from build123d import *

# Parameters (mm, degrees)
CYLINDER_R     = 10
CYLINDER_DEPTH = 40
BOX_W          = 30
BOX_H          = 24
BOX_DEPTH      = 40


with BuildPart() as cilindro:
    # Cylinder → Cylinder (new body)
    with BuildSketch(Plane(origin=(11, 12, -16), x_dir=(1, 0, 0), z_dir=(0, 0, 1))):
        Circle(CYLINDER_R)
    extrude(amount=CYLINDER_DEPTH)


with BuildPart() as cut:
    # Box → Box (new body)
    with BuildSketch(Plane(origin=(-1, 0, -12), x_dir=(1, 0, 0), z_dir=(0, 0, 1))):
        with Locations((15, 12)):
            Rectangle(BOX_W, BOX_H)
    extrude(amount=BOX_DEPTH)

    # Cut: cut Cilindro
    add(cilindro.part, mode=Mode.SUBTRACT)


solid = cut.part
Could you check a few things on this model? Use its own coordinates, in mm. A direction names the side the tool comes from. Give positions to 0.01 mm unless a question says otherwise; leave off trailing zeros. Order: outer loops, then holes, each group sorted by start corner. A loop starts at its lowest first (then second) coordinate and runs counter-clockwise, first axis right, second up. Notation, with made-up numbers: M 36.5,35.25 L 68.5,35.25 A22 ccw 68.5,47.25 Z; hole C 67,-39 d5. An arc over 180 degrees is marked long. One line per question, with ' | ' between items.
1. I want a section at C-C (x = 3). List the corners of the cut face in (y, z) for me, and give its area (3 significant figures).
Results:
outline: M 0,-12 L 6,-12 L 6,24 L 18,24 L 18,-12 L 24,-12 L 24,28 L 0,28 Z | area: 528 mm²
2. For faces 4 (the face through (11, 12, 24)), 5 (the face through (20, 18, -12)), which set-ups out of +Z, -Z, +X, -X, +Y, -Y let a thin tool reach every point of the face, with its end or its side?
Results:
face 4: -Z | face 5: -Z, +X, -X, +Y, -Y
3. We'd pull the mould along X, two halves only. Please class faces 1 (the face through (29, 12, 8)), 2 (the face through (14, 12, 28)), 3 (the face through (3, 6, 6)): +X half, -X half, draft (parallel to the pull), parting line (faces both ways), or undercut.
Results:
face 1: +X half | face 2: draft | face 3: undercut
4. I want a section at B-B (y = 12). List the corners of the cut face in (x, z) for me.
Results:
outline: M -1,-12 L 1,-12 L 1,24 L 21,24 L 21,-12 L 29,-12 L 29,28 L -1,28 Z
5. I want a section at A-A (z = 4.5). List the corners of the cut face in (x, y) for me.
Results:
outline: M -1,0 L 29,0 L 29,24 L -1,24 Z; hole C 11,12 d20
6. I'm going to push a flat-ended pin straight in: pin 1 (1.5 mm diameter, centred on x = 9.5, y = 17, fed in from -Z). Where does the tip first touch, or does it pass through?
Results:
pin 1: z = 24
7. If I drill on line 1 (Y direction, x = 11.25, z = 5.5); line 2 (X direction, y = 12, z = 11); line 3 (X direction, y = 5.75, z = -6), over which ranges is the centre line in solid material (lowest first)?
Results:
line 1: 0 to 2, 22 to 24 | line 2: -1 to 1, 21 to 29 | line 3: -1 to 3.19, 18.81 to 29
